from build123d import *

# Parameters (mm, degrees)
ESTRUSIONE_ESTRUSIONE1_DEPTH  = 25
RACCORDO1_R                   = 2
RACCORDO2_R                   = 2
TAGLIO_ESTRUSIONE5_DEPTH      = 1
TAGLIO_ESTRUSIONE5_DEPTH_BACK = 56
SCHIZZO8_9_R                  = 1.5
SCHIZZO8_9_R_2                = 4
TAGLIO_ESTRUSIONE6_DEPTH      = 1
TAGLIO_ESTRUSIONE6_DEPTH_BACK = 56
SCHIZZO11_R                   = 4
SCHIZZO11_R_2                 = 1.5
TAGLIO_ESTRUSIONE7_DEPTH      = 64
TAGLIO_ESTRUSIONE7_DEPTH_BACK = 3


with BuildPart() as part:
    # Schizzo4 → Estrusione-Estrusione1 (new body)
    with BuildSketch(Plane.XY):
        Polygon((-48.72252025, 30.495594714), (-48.72252025, -34.504405286), (6.27747975, -34.504405286), (6.27747975, 30.495594714), (4.27747975, 30.495594714), (4.27747975, -32.504405286), (-46.72252025, -32.504405286), (-46.72252025, 30.495594714), align=None)
    extrude(amount=ESTRUSIONE_ESTRUSIONE1_DEPTH)

    # Raccordo1
    raccordo1_edges = [part.edges().sort_by_distance(p)[0] for p in [
        (6.27747975, -34.504405286, 12.5),
    ]]
    fillet(raccordo1_edges, radius=RACCORDO1_R)

    # Raccordo2
    raccordo2_edges = [part.edges().sort_by_distance(p)[0] for p in [
        (-48.72252025, -34.504405286, 12.5),
    ]]
    fillet(raccordo2_edges, radius=RACCORDO2_R)

    # Schizzo8 → Taglio-Estrusione5 (cut, two sides)
    with BuildSketch(Plane(origin=(6.27747975, 0, 0), x_dir=(0, 0, -1), z_dir=(1, 0, 0))) as taglio_estrusione5_sk:
        with BuildLine():
            Line((0, 30.495594714), (-12.5, 30.495594714))
            ThreePointArc((-12.5, 30.495594714), (-3.661165235, 26.834429478), (0, 17.995594714))
            Line((0, 17.995594714), (0, 30.495594714))
        make_face()
        with BuildLine():
            Line((-12.5, 30.495594714), (-25, 30.495594714))
            Line((-25, 30.495594714), (-25, 17.995594714))
            ThreePointArc((-25, 17.995594714), (-21.338834765, 26.834429478), (-12.5, 30.495594714))
        make_face()
    extrude(amount=TAGLIO_ESTRUSIONE5_DEPTH, mode=Mode.SUBTRACT)
    extrude(taglio_estrusione5_sk.sketch, amount=-TAGLIO_ESTRUSIONE5_DEPTH_BACK, mode=Mode.SUBTRACT)

    # Schizzo8<9> → Taglio-Estrusione6 (cut, two sides)
    with BuildSketch(Plane(origin=(6.27747975, 0, 0), x_dir=(0, 0, -1), z_dir=(1, 0, 0))) as taglio_estrusione6_sk:
        with Locations((-19.5, 17.995594714)):
            Circle(SCHIZZO8_9_R)
        with Locations((-12.5, 17.995594714)):
            Circle(SCHIZZO8_9_R_2)
        with Locations((-12.5, 24.995594714)):
            Circle(SCHIZZO8_9_R)
        with Locations((-5.5, 17.995594714)):
            Circle(SCHIZZO8_9_R)
        with Locations((-12.5, 10.995594714)):
            Circle(SCHIZZO8_9_R)
        with Locations((-12.5, 0.995594714)):
            Circle(SCHIZZO8_9_R)
        with Locations((-12.5, -16.004405286)):
            Circle(SCHIZZO8_9_R)
    extrude(amount=TAGLIO_ESTRUSIONE6_DEPTH, mode=Mode.SUBTRACT)
    extrude(taglio_estrusione6_sk.sketch, amount=-TAGLIO_ESTRUSIONE6_DEPTH_BACK, mode=Mode.SUBTRACT)

    # Schizzo11 → Taglio-Estrusione7 (cut, two sides)
    with BuildSketch(Plane(origin=(0, -32.504405286, 0), x_dir=(1, 0, 0), z_dir=(0, 1, 0))) as taglio_estrusione7_sk:
        with Locations((-21.22252025, -12.5)):
            Circle(SCHIZZO11_R)
        with Locations((-21.22252025, -5.5)):
            Circle(SCHIZZO11_R_2)
        with Locations((-28.22252025, -12.5)):
            Circle(SCHIZZO11_R_2)
        with Locations((-21.22252025, -19.5)):
            Circle(SCHIZZO11_R_2)
        with Locations((-14.22252025, -12.5)):
            Circle(SCHIZZO11_R_2)
        with Locations((-2.22252025, -12.5)):
            Circle(SCHIZZO11_R_2)
        with Locations((-40.22252025, -12.5)):
            Circle(SCHIZZO11_R_2)
    extrude(amount=TAGLIO_ESTRUSIONE7_DEPTH, mode=Mode.SUBTRACT)
    extrude(taglio_estrusione7_sk.sketch, amount=-TAGLIO_ESTRUSIONE7_DEPTH_BACK, mode=Mode.SUBTRACT)


solid = part.part
The listing builds one solid part. Answer for the finished solid, in the listing's coordinates (mm). A direction names the side the tool comes from. Coordinates: 2 decimals unless noted, no trailing zeros. Order: outer loops, then holes, each group sorted by start corner. A loop starts at its lowest first (then second) coordinate and runs counter-clockwise, first axis right, second up. Notation, with made-up numbers: M 27,89.25 L 81,89.25 A33 cw 81,121.25 Z; hole C 22.25,1.5 d3. An arc over 180 degrees is marked long. Use CSV: the item, a comma, the result in double quotes.
Q1. Section B-B (z = 19.5) is taken. Determine the outline of the cut face in (x, y).
Here are the results:
outline,"M -48.72,-32.5 A2 ccw -46.72,-34.5 L -22.72,-34.5 L -22.72,-32.5 L -46.72,-32.5 L -46.72,16.5 L -48.72,16.5 Z; M -48.72,19.5 L -46.72,19.5 L -46.72,28.35 L -48.72,28.35 Z; M -19.72,-34.5 L 4.28,-34.5 A2 ccw 6.28,-32.5 L 6.28,16.5 L 4.28,16.5 L 4.28,-32.5 L -19.72,-32.5 Z; M 4.28,19.5 L 6.28,19.5 L 6.28,28.35 L 4.28,28.35 Z"
Q2. Straight lines are drawn through the part: L1, parallel to X at y = -23, z = 14.75; L2, parallel to Z at x = 4.5, y = 19; L3, parallel to X at y = -33.6, z = 12.5. For each, find the intervals that lie inside material, in ascending order.
Here are the results:
L1,"-48.72 to -46.72, 4.28 to 6.28"
L2,"0.04 to 4.39, 6.61 to 8.63, 16.37 to 18.39, 20.61 to 24.96"
L3,"-48.4 to -41.72, -38.72 to -29.72, -26.72 to -25.22, -17.22 to -15.72, -12.72 to -3.72, -0.72 to 5.95"
Q3. Section C-C (x = -32.5) is taken. Determine the outline of the cut face in (y, z).
Here are the results:
outline,"M -34.5,0 L -32.5,0 L -32.5,25 L -34.5,25 Z"
Q4. Given pin 1 Ø5 at (y, z) = (18, 12.5) entering from -X; pin 2 Ø4 at (x, z) = (-21.22, 19.5) entering from +Y, each flat-ended and moving along its own axis, determine where each tip first touches the part or whether it passes through.
Here are the results:
pin 1,"through"
pin 2,"y = -32.5"
Q5. A tool of negligible diameter and unlimited length cuts with its end or side. For faces 4 (the flat face through (-46.723, -1, 12)), 5 (the cylindrical face through (5.68, -33.93, 12.68)), from which of +Z, -Z, +X, -X, +Y, -Y can it reach the whole face along a straight path? Write none if from no direction.
Here are the results:
face 4,"+Z, -Z, +Y"
face 5,"+Z, -Z, +X, -Y"
Q6. Section A-A (x = -24) is taken. Determine the outline of the cut face in (y, z), then the cut area to 3 significant figures.
Here are the results:
outline,"M -34.5,0 L -32.5,0 L -32.5,9.62 L -34.5,9.62 Z; M -34.5,15.38 L -32.5,15.38 L -32.5,25 L -34.5,25 Z"
area,"38.5 mm2"
Q7. Determine the mould class of faces 1 (the flat face through (-26.5, -32.504, 12.3)), 2 (the cylindrical face through (5, 18, 21)), 3 (the cylindrical face through (-26.79, -33.49, 12.05)) for opening direction Y: pulls with the +Y half, pulls with the -Y half, needs draft (parallel to the pull), parting line crosses it, or undercut.
Here are the results:
face 1,"pulls with the +Y half"
face 2,"undercut"
face 3,"needs draft"
